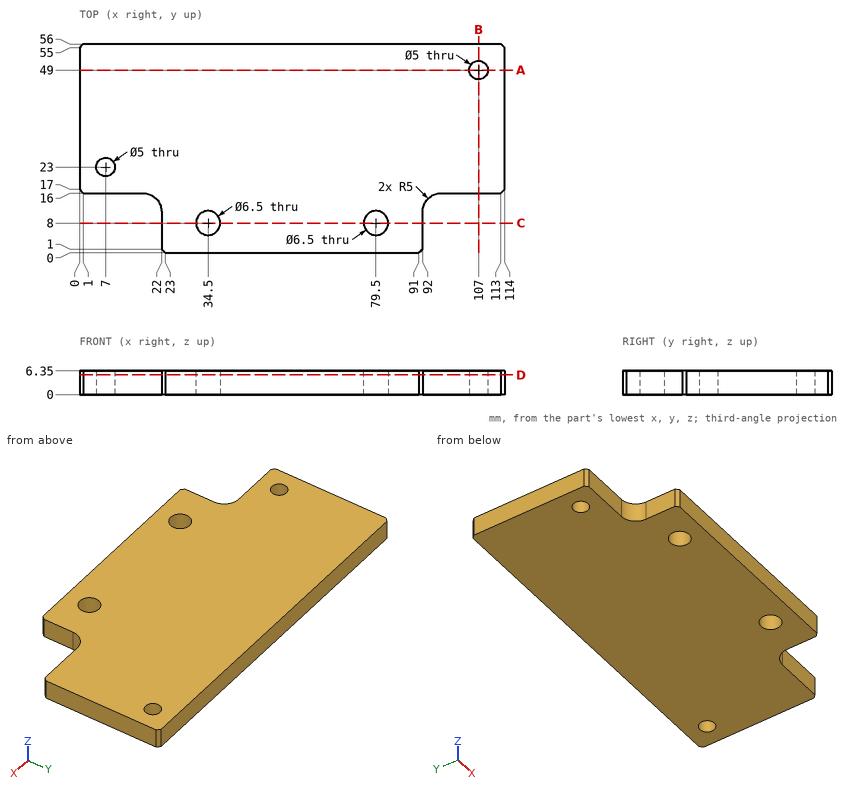
Geometry check sheet. Reference: drawing and pictorial views, mm from the part's lowest x, y, z. Give positions to 0.01 mm unless a question says otherwise; leave off trailing zeros. Loops run counter-clockwise (first coordinate to the right, second up) from the corner with the lowest first, then second, coordinate; pieces in that order, holes last.
1. Section check A-A, the plane y = 49. Enter the section's corners in (x, z), then the cut area to 3 significant figures.
2. Thickness scan on line 1 (Y direction, x = 79.5, z = 4.25); line 2 (Y direction, x = 7, z = 4.5); line 3 (X direction, y = 51, z = 2.5). Record the ranges inside material, lowest first.
3. Section check B-B, the plane x = 107. Enter the section's corners in (y, z).
4. Section check D-D, the plane z = 5.25. Enter the section's corners in (x, y), then the cut area to 3 significant figures.
5. Section check C-C, the plane y = 8. Enter the section's corners in (x, z).
6. Go/stop test with flat-tipped pins: pin 1 Ø1 at (y, z) = (39, 2.5) entering from -X; pin 2 Ø3 at (y, z) = (5, 2) entering from +X; pin 3 Ø6 at (x, y) = (34.5, 8) entering from +Z. Record where each tip stops, or that it passes through.
Geometry says:
1. outline: (0, 0) - (104.5, 0) - (104.5, 6.35) - (0, 6.35) - close; (109.5, 0) - (114, 0) - (114, 6.35) - (109.5, 6.35) - close
1. area: 692 mm2
2. line 1: y = 0 to 4.75, 11.25 to 56
2. line 2: y = 16 to 20.5, 25.5 to 56
2. line 3: x = 0 to 105.5, 108.5 to 114
3. outline: (16, 0) - (46.5, 0) - (46.5, 6.35) - (16, 6.35) - close; (51.5, 0) - (56, 0) - (56, 6.35) - (51.5, 6.35) - close
4. outline: (0, 17) - (1, 16) - (17, 16) arc R5 cw to (22, 11) - (22, 1) - (23, 0) - (91, 0) - (92, 1) - (92, 11) arc R5 cw to (97, 16) - (113, 16) - (114, 17) - (114, 55) - (113, 56) - (1, 56) - (0, 55) - close; hole circle Ø5 at (7, 23); hole circle Ø6.5 at (34.5, 8); hole circle Ø6.5 at (79.5, 8); hole circle Ø5 at (107, 49)
4. area: 5,580 mm2
5. outline: (22, 0) - (31.25, 0) - (31.25, 6.35) - (22, 6.35) - close; (37.75, 0) - (76.25, 0) - (76.25, 6.35) - (37.75, 6.35) - close; (82.75, 0) - (92, 0) - (92, 6.35) - (82.75, 6.35) - close
6. pin 1: stops at x = 0
6. pin 2: stops at x = 92
6. pin 3: passes through
